Here's how the part is built. I have some questions about the finished solid (model axes, mm). Face numbers are marked on the shaded views. A direction names the side the tool comes from. Give positions to 0.01 mm unless a question says otherwise; leave off trailing zeros. Write each loop counter-clockwise with the first axis right and the second up, starting at its lowest first coordinate (ties: lowest second). Pieces come first, ordered by that corner, then holes. Notation, with made-up numbers: M -32.5,-27.75 L 25.5,-27.75 A4 ccw 25.5,-20.75 Z; hole C 21,59.25 d10. An arc over 180 degrees is marked long. Answer as CSV lines item,"result". Start each with the question number.
Q1. On a 3-axis mill with a long thin cutter (end or side, diameter ignored), from which of +Z, -Z, +X, -X, +Y, -Y can I reach the whole of each face in a straight line? I mean the marked faces 5, 6, 7 and 8. Say none if no direction works.
Q2. Suppose I cut it at C-C (x = 0). Write out the boundary of the cut face in (y, z).
Q3. If I drill on line 1 along Z through (x, y) = (2.5, 1); line 2 along Z through (x, y) = (0.75, 3.75); line 3 along Y through (x, z) = (0, 7.25), over which ranges is the centre line in solid material (lowest first)?
Q4. Suppose I cut it at A-A (z = -2). Write out the boundary of the cut face in (x, y).
Q5. For pin 1 (1 mm diameter, centred on y = -1, z = 7, fed in from -X); pin 2 (0.9 mm diameter, centred on y = 3, z = -3, fed in from +X); pin 3 (1.4 mm diameter, centred on y = 3, z = -2.5, fed in from -X); pin 4 (0.9 mm diameter, centred on x = 0, y = 0, fed in from +Z), each with a flat end and sliding along its axis, tell me the tip position at first contact or that it passes through.
Q6. Thinking about a two-plate mould opening in Z: for the marked faces 1, 2, 3 and 4, which applies, +Z half, -Z half, draft (parallel to the pull), parting line (faces both ways), or undercut?
Q7. Suppose I cut it at D-D (z = -0.25). Write out the boundary of the cut face in (x, y), then the cut area to 3 significant figures.
Q8. Suppose I cut it at B-B (y = 0). Write out the boundary of the cut face in (x, z).
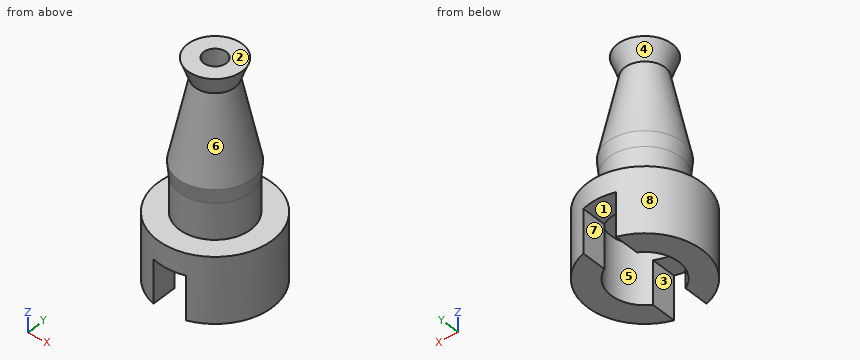
```python
from build123d import *

# Parameters (mm, degrees)
SKETCH001_R          = 2.3495
POCKET_DEPTH         = 4.064
SKETCH002_R          = 0.7874
POCKET001_DEPTH      = 15.073
SKETCH003_W          = 2.286
SKETCH003_H          = 5.08
POCKET002_DEPTH      = 5.0038
POCKET002_DEPTH_BACK = -99.9998


with BuildPart() as part:
    # Sketch → Revolution (revolve)
    with BuildSketch(Plane.XZ):
        Polygon((2.5, 0), (4, 0), (4, -4.572), (0, -4.572), (0, 0), (0, 10.5), (1.9, 10.5), (1.4, 9.15), (2.6, 3.5), (2.5, 2.5), align=None)
    revolve(axis=Axis((0, 0, 0), (0, 0, 1)))

    # Sketch001 (on Face5 of Revolution) → Pocket (cut)
    with BuildSketch(Plane(origin=(0, 0, -4.572), x_dir=(1, 0, 0), z_dir=(0, 0, -1))):
        Circle(SKETCH001_R)
    extrude(amount=-POCKET_DEPTH, mode=Mode.SUBTRACT)

    # Sketch002 (on Face6 of Pocket) → Pocket001 (cut, through all)
    with BuildSketch(Plane(origin=(0, 0, 10.5), x_dir=(-1, 0, 0), z_dir=(0, 0, 1))):
        Circle(SKETCH002_R)
    extrude(amount=-POCKET001_DEPTH, mode=Mode.SUBTRACT)

    # Sketch003 → Pocket002 (cut, two sides)
    with BuildSketch(Plane.XZ) as pocket002_sk:
        with Locations((0, -4.064)):
            Rectangle(SKETCH003_W, SKETCH003_H)
    extrude(amount=-POCKET002_DEPTH, mode=Mode.SUBTRACT)
    extrude(pocket002_sk.sketch, amount=-POCKET002_DEPTH_BACK, mode=Mode.SUBTRACT)


solid = part.part
```
Resolved:
1,face 5,"-Z"
1,face 6,"none"
1,face 7,"-Z, +Y, -Y"
1,face 8,"+Z, -Z"
2,outline,"M -4,-1.52 L -2.35,-1.52 L -2.35,-0.51 L -0.79,-0.51 L -0.79,10.5 L -1.9,10.5 L -1.4,9.15 L -2.6,3.5 L -2.5,2.5 L -2.5,0 L -4,0 Z; M 0.79,-0.51 L 2.35,-0.51 L 2.35,-1.52 L 4,-1.52 L 4,0 L 2.5,0 L 2.5,2.5 L 2.6,3.5 L 1.4,9.15 L 1.9,10.5 L 0.79,10.5 Z"
3,line 1,"-4.57 to 0"
3,line 2,"-1.52 to 0"
3,line 3,"-1.8 to -0.79, 0.79 to 1.8"
4,outline,"M -1.14,-3.83 L -1.14,-2.05 A2.35 cw -1.14,2.05 L -1.14,3.83 A4 ccw Z; M 1.14,-3.83 A4 ccw 1.14,3.83 L 1.14,2.05 A2.35 cw 1.14,-2.05 Z"
5,pin 1,"x = -1.82"
5,pin 2,"x = 3.08"
5,pin 3,"x = -3.27"
5,pin 4,"through"
6,face 1,"-Z half"
6,face 2,"+Z half"
6,face 3,"draft"
6,face 4,"undercut"
7,outline,"C 0,0 d8; hole C 0,0 d1.57"
7,area,"48.3 mm^2"
8,outline,"M -4,-4.57 L -2.35,-4.57 L -2.35,-0.51 L -0.79,-0.51 L -0.79,10.5 L -1.9,10.5 L -1.4,9.15 L -2.6,3.5 L -2.5,2.5 L -2.5,0 L -4,0 Z; M 0.79,-0.51 L 2.35,-0.51 L 2.35,-4.57 L 4,-4.57 L 4,0 L 2.5,0 L 2.5,2.5 L 2.6,3.5 L 1.4,9.15 L 1.9,10.5 L 0.79,10.5 Z"
